Autodesk Inventor part; units mm, degrees
ref_plane "YZ Plane" through (0, 0, 0) normal (1, 0, 0) x (0, 1, 0)
ref_plane "XZ Plane" through (0, 0, 0) normal (0, 1, 0) x (-1, 0, 0)
ref_plane "XY Plane" through (0, 0, 0) normal (0, 0, 1) x (1, 0, 0)
sketch "Sketch1" plane through (0, 0, 0) normal (0, 1, 0) x (-1, 0, 0)
  line L0 (0, 0) -> (0, -312.648) construction
  line L1 (5, 0) -> (5, -312.648)
  line L2 (-5, -312.648) -> (-5, 0)
  arc A0 (5, 0) -> (-5, 0) centre (0, 0) ccw
  arc A1 (-5, -312.648) -> (5, -312.648) centre (0, -312.648) ccw
  circle A2 centre (0, 0) radius 1.65
  circle A3 centre (0, -312.648) radius 1.65
  circle A4 centre (0, -42.6) radius 1.65
  circle A5 centre (0, -254.274) radius 1.65
  arc A6 (5, -254.274) -> (5, -42.6) centre (-585.5917, -148.437) ccw
  arc A7 (-5, -254.274) -> (-5, -42.6) centre (-595.5917, -148.437) ccw
  point P0 (0, -156.324)
  dimension "d0" = 3.3
  dimension "d1" = 3.3
  dimension "d2" = 10
  dimension "d3" = 312.648
  dimension "d10" = 3.3
  dimension "d11" = 42.6
  dimension "d12" = 3.3
  dimension "d13" = 254.274
  dimension "d16" = 600
  dimension "d17" = 600
extrude "Extrusion1" add sketch "Sketch1" along normal blind 3 contours L1 A1 L2 A7 A0 | A6 L1
sketch "Sketch2" plane through (0, 3, 0) normal (0, 1, 0) x (1, 0, 0)
  line L0 (-83.1437, 348.5388) -> (78.2815, 348.5388)
  line L1 (78.2815, 348.5388) -> (78.2815, -47.0064)
  line L2 (78.2815, -47.0064) -> (-83.1437, -47.0064)
  line L3 (-83.1437, -47.0064) -> (-83.1437, 348.5388)
  line L4 (-31.117, 331.0778) -> (31.6, 331.0778)
  line L5 (31.6, 331.0778) -> (31.6, 150.7662)
  line L6 (31.6, 150.7662) -> (-31.117, 150.7662)
  line L7 (-31.117, 150.7662) -> (-31.117, 331.0778)
  point P0 (0, 0)
extrude "Extrusion2" cut sketch "Sketch2" against normal blind 10 contours L4 L5 L6 L7
properties part number "Part_5_p1"
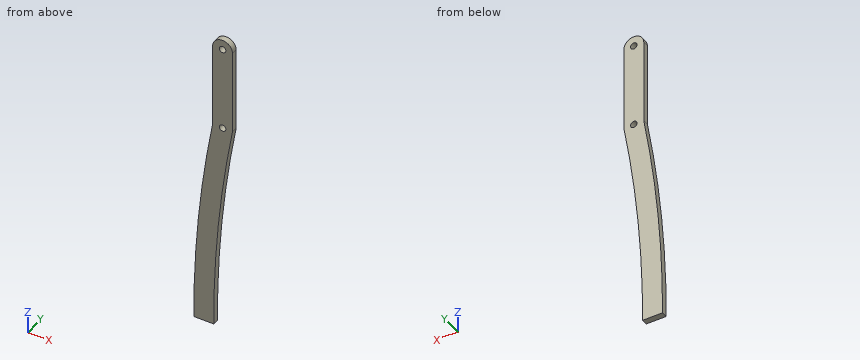
Work out the finished part from the listing and answer in its coordinate system (mm). Give positions to 0.01 mm unless a question says otherwise; leave off trailing zeros. Loops run counter-clockwise (first coordinate to the right, second up) from the corner with the lowest first, then second, coordinate; pieces in that order, holes last. Notation, with made-up numbers: (46, 15) -> (79, 15) arc R24 ccw to (79, 26) -> close; hole circle Ø10 at (-35.5, 76.5). An arc over 180 degrees is marked (long way). Use a Markdown table: item, result. Add a question column.
1. Section A-A on y = 0.5 is taken. Determine the outline of the cut face in (x, z), and give its area (3 significant figures).
2. Find the intervals of material crossed by probe 1 along X at (y, z) = (2.3, -7); probe 2 along X at (y, z) = (2.8, -117); probe 3 along Z at (x, y) = (-4.5, 1.6), in increasing order.
3. Flat-ended cylindrical pins translate along their axes: pin 1 Ø2.5 at (x, z) = (0, 0) entering from +Y; pin 2 Ø0.9 at (y, z) = (2, -18.5) entering from -X; pin 3 Ø1.5 at (y, z) = (1, -102) entering from +X; pin 4 Ø1.5 at (y, z) = (1, -66) entering from +X. Find the tip coordinate at first contact, or state that the pin passes through.
4. Section D-D on z = -81 is taken. Determine the outline of the cut face in (x, y), and give its area (3 significant figures).
5. Section B-B on x = 0 is taken. Determine the outline of the cut face in (y, z).
Results below:
| question | item | result |
|---|---|---|
| 1 | outline | (-14.4, -150.77) -> (-4.4, -150.77) arc R600 cw to (5, -42.6) -> (5, 0) arc R5 ccw to (-5, 0) -> (-5, -42.6) arc R600 ccw to start; hole circle Ø3.3 at (0, -42.6); hole circle Ø3.3 at (0, 0) |
| 1 | area | 1,530 mm^2 |
| 2 | probe 1 | x = -5 to 5 |
| 2 | probe 2 | x = -13.58 to -3.58 |
| 2 | probe 3 | z = -150.77 to 2.18 |
| 3 | pin 1 | passes through |
| 3 | pin 2 | stops at x = -5 |
| 3 | pin 3 | stops at x = -2.55 |
| 3 | pin 4 | stops at x = 1.39 |
| 4 | outline | (-10.61, 0) -> (-0.61, 0) -> (-0.61, 3) -> (-10.61, 3) -> close |
| 4 | area | 30.0 mm^2 |
| 5 | outline | (0, -75.84) -> (3, -75.84) -> (3, -44.25) -> (0, -44.25) -> close; (0, -40.95) -> (3, -40.95) -> (3, -1.65) -> (0, -1.65) -> close; (0, 1.65) -> (3, 1.65) -> (3, 5) -> (0, 5) -> close |
